Work out the finished part from the listing and answer in its coordinate system (mm). Round coordinates to 2 decimals unless told otherwise and drop trailing zeros. Loops run counter-clockwise (first coordinate to the right, second up) from the corner with the lowest first, then second, coordinate; pieces in that order, holes last. Notation, with made-up numbers: (88, 38.25) -> (144, 38.25) arc R21 cw to (144, 64.25) -> close; hole circle Ø6 at (13.5, -22.75). An arc over 180 degrees is marked (long way). Use CSV: the item, a comma, the result in double quotes. Start each with the question number.
from build123d import *

# Parameters (mm, degrees)
SKETCH_1_R      = 9
SKETCH_1_R_2    = 2
EXTRUDE_1_DEPTH = 1.3
SKETCH_2_R      = 4
SKETCH_2_R_2    = 2
EXTRUDE_2_DEPTH = 0.2


with BuildPart() as part:
    # Эскиз1 → Бобышка-Вытянуть1 (new body)
    with BuildSketch(Plane.XY):
        Circle(SKETCH_1_R)
        Circle(SKETCH_1_R_2, mode=Mode.SUBTRACT)
    extrude(amount=EXTRUDE_1_DEPTH)

    # Эскиз2 → Бобышка-Вытянуть2 (add)
    with BuildSketch(Plane.XY.offset(1.3)):
        Circle(SKETCH_2_R)
        Circle(SKETCH_2_R_2, mode=Mode.SUBTRACT)
    extrude(amount=EXTRUDE_2_DEPTH)

    # Эскиз3 → Вырез-Повернуть1 (revolve, cut)
    with BuildSketch(Plane(origin=(0, 0, 0), x_dir=(1, 0, 0), z_dir=(0, 1, 0))):
        Polygon((-4, -1.3), (-9, -0.65), (-9, -1.3), align=None)
    revolve(axis=Axis((0, 0, 0), (0, 0, 1)), mode=Mode.SUBTRACT)


solid = part.part
Q1. Straight lines are drawn through the part: line 1 (Y direction, x = 0, z = 0.55); line 2 (Y direction, x = 1.75, z = 0.6); line 3 (Z direction, x = 6.5, y = 5.5). For each, find the intervals that lie inside material, in ascending order. Write a range as from..to.
Q2. Section A-A, the plane y = 0 is taken. Write down the section's boundary in (x, z), and give its area (4 significant figures).
Q3. Each of these flat-tipped pins is pushed along its axis until it touches: pin 1 (6.5 mm diameter, centred on x = 0, y = 0, fed in from +Z); pin 2 (3 mm diameter, centred on x = 0, y = 6, fed in from +Z) (3 decimals); pin 3 (1 mm diameter, centred on x = -7, y = 5, fed in from +Z). Where does it stop, or does it pass through?
Q4. For a pull along Y with two mould halves and no side action, classify faces 1 (the cylindrical face through (0, -2, 1)), 2 (the cylindrical face through (-1.172, 8.923, 0.32)), 3 (the flat face through (2, -2, 0)) as pulls with the +Y half, pulls with the -Y half, needs draft (parallel to the pull), parting line crosses it, or undercut.
Report:
1,line 1,"y = -9..-2, 2..9"
1,line 2,"y = -8.83..-0.97, 0.97..8.83"
1,line 3,"z = 0..0.71"
2,outline,"(-9, 0) -> (-2, 0) -> (-2, 1.5) -> (-4, 1.5) -> (-4, 1.3) -> (-9, 0.65) -> close; (2, 0) -> (9, 0) -> (9, 0.65) -> (4, 1.3) -> (4, 1.5) -> (2, 1.5) -> close"
2,area,"15.75 mm²"
3,pin 1,"stops at z = 1.5"
3,pin 2,"stops at z = 1.235"
3,pin 3,"stops at z = 0.77"
4,face 1,"undercut"
4,face 2,"parting line crosses it"
4,face 3,"needs draft"
